Here's how the part is built. I have some questions about the finished solid (model axes, mm). A direction names the side the tool comes from. Round coordinates to 2 decimals unless told otherwise and drop trailing zeros. Loops run counter-clockwise (first coordinate to the right, second up) from the corner with the lowest first, then second, coordinate; pieces in that order, holes last. Notation, with made-up numbers: M -30.75,50 L 22.25,50 A9 ccw 22.25,60 Z; hole C -24,-38 d5. An arc over 180 degrees is marked long. Answer as a JSON object with one key per item and string values.
from build123d import *

# Parameters (mm, degrees)
SKETCH_1_W           = 15
SKETCH_1_H           = 15
EXTRUDE_1_DEPTH      = 4
EXTRUDE_2_DEPTH      = 5.5
EXTRUDE_2_DEPTH_BACK = 9.5
SKETCH_2_R           = 4.25
SKETCH_5_R           = 3
CUT_EXTRUDE_3_DEPTH  = 19.371173071
SKETCH_3_R           = 1
CUT_EXTRUDE_1_DEPTH  = 15.239030866
SKETCH_4_R           = 2
CUT_EXTRUDE_2_DEPTH  = 1
SKETCH_6_W           = 1
SKETCH_6_H           = 2.949438202
CUT_EXTRUDE_4_DEPTH  = 3.5


with BuildPart() as part:
    # 草图1 → 拉伸1 (new body)
    with BuildSketch(Plane(origin=(0, 0, 0), x_dir=(1, 0, 0), z_dir=(0, 1, 0))):
        Rectangle(SKETCH_1_W, SKETCH_1_H)
    extrude(amount=EXTRUDE_1_DEPTH)

    # 草图2 → 拉伸2 (add, two sides: drawn at the far end of the back side and taken through both)
    with BuildSketch(Plane(origin=(0, 4, 0), x_dir=(-1, 0, 0), z_dir=(0, 1, 0)).offset(-EXTRUDE_2_DEPTH_BACK)):
        with Locations(Location((0, 0, 0), (0, 0, 90))):
            Circle(SKETCH_2_R)
    extrude(amount=EXTRUDE_2_DEPTH + EXTRUDE_2_DEPTH_BACK)

    # 草图5 → 切除-拉伸3 (cut, through all)
    with BuildSketch(Plane.XZ.offset(5.5)):
        with Locations(Location((0, 0, 0), (0, 0, 270))):
            Circle(SKETCH_5_R)
    extrude(amount=-CUT_EXTRUDE_3_DEPTH, mode=Mode.SUBTRACT)

    # 草图3 → 切除-拉伸1 (cut, through all)
    with BuildSketch(Plane(origin=(0, 4, 0), x_dir=(-1, 0, 0), z_dir=(0, 1, 0))):
        with Locations(Location((5, -5, 0), (0, 0, 90))):
            Circle(SKETCH_3_R)
        with Locations(Location((-5, 5, 0), (0, 0, 90))):
            Circle(SKETCH_3_R)
    extrude(amount=-CUT_EXTRUDE_1_DEPTH, mode=Mode.SUBTRACT)

    # 草图4 → 切除-拉伸2 (cut)
    with BuildSketch(Plane(origin=(0, 4, 0), x_dir=(-1, 0, 0), z_dir=(0, 1, 0))):
        with Locations(Location((5, -5, 0), (0, 0, 90))):
            Circle(SKETCH_4_R)
        with Locations(Location((-5, 5, 0), (0, 0, 90))):
            Circle(SKETCH_4_R)
    extrude(amount=-CUT_EXTRUDE_2_DEPTH, mode=Mode.SUBTRACT)

    # 草图6 → 切除-拉伸4 (cut)
    with BuildSketch(Plane(origin=(0, 9.5, 0), x_dir=(-1, 0, 0), z_dir=(0, 1, 0))):
        with Locations((0, 3.651685393)):
            Rectangle(SKETCH_6_W, SKETCH_6_H)
    extrude(amount=-CUT_EXTRUDE_4_DEPTH, mode=Mode.SUBTRACT)


solid = part.part
Item 1: Please list where these lines run through material, in increasing order: probe 1 along X at (y, z) = (3.6, -5); probe 2 along Z at (x, y) = (0, 2.25); probe 3 along X at (y, z) = (1.8, -5). Write a range as from..to.
Resolved:
{"probe 1": "-7.5..-7, -3..7.5", "probe 2": "-7.5..-3, 3..7.5", "probe 3": "-7.5..-6, -4..7.5"}
Item 2: If we mould it in two halves opening along X, with no side actions, what happens to faces 1 (the face through (5.088, 3.507, 3.002)), 2 (the face through (7.5, 2, 0)), 3 (the face through (-1, -5.5, -3)), 4 (the face through (-0.5, 8, 4))? For each: pulls with the +X half, pulls with the -X half, needs draft (parallel to the pull), parting line crosses it, or undercut.
Resolved:
{"face 1": "undercut", "face 2": "pulls with the +X half", "face 3": "needs draft", "face 4": "undercut"}
Item 3: I want a section at B-B, the plane y = 2.5. Please give me the cut outline in (x, z), then the cut area to 3 significant figures.
Resolved:
{"outline": "M -7.5,-7.5 L 7.5,-7.5 L 7.5,7.5 L -7.5,7.5 Z; hole C -5,-5 d2; hole C 0,0 d6; hole C 5,5 d2", "area": "190 mm²"}
Item 4: I'm going to push flat-ended pins straight in: pin 1 Ø1 at (x, y) = (1, -2) entering from +Z; pin 2 Ø1.5 at (y, z) = (7, 3) entering from +X; pin 3 Ø5 at (x, z) = (-5.5, 5.5) entering from -Y; pin 4 Ø8 at (x, z) = (0, 0) entering from -Y. Where does each tip first touch, or does it pass through?
Resolved:
{"pin 1": "z = 4.22", "pin 2": "x = 3.61", "pin 3": "y = 0", "pin 4": "y = -5.5"}
Item 5: I want a section at A-A, the plane x = 0. Please give me the cut outline in (y, z).
Resolved:
{"outline": "M -5.5,-4.25 L 0,-4.25 L 0,-7.5 L 4,-7.5 L 4,-4.25 L 9.5,-4.25 L 9.5,-3 L -5.5,-3 Z; M -5.5,3 L 6,3 L 6,4.25 L 4,4.25 L 4,7.5 L 0,7.5 L 0,4.25 L -5.5,4.25 Z"}
Item 6: I want a section at C-C, the plane z = -5. Please give me the cut outline in (x, y).
Resolved:
{"outline": "M -7.5,0 L -6,0 L -6,3 L -7,3 L -7,4 L -7.5,4 Z; M -4,0 L 7.5,0 L 7.5,4 L -3,4 L -3,3 L -4,3 Z"}
Item 7: I want a section at D-D, the plane x = 5. Please give me the cut outline in (y, z).
Resolved:
{"outline": "M 0,-7.5 L 4,-7.5 L 4,3 L 3,3 L 3,4 L 0,4 Z; M 0,6 L 3,6 L 3,7 L 4,7 L 4,7.5 L 0,7.5 Z"}
Item 8: On a 3-axis mill with a long thin cutter (end or side, diameter ignored), from which of +Z, -Z, +X, -X, +Y, -Y can I reach the whole of each face in a straight line? I mean faces 5 (the face through (3, 9.5, -1)), 6 (the face through (4.214, -2.788, -0.553)), 7 (the face through (0, 6, 4)), 8 (the face through (4.214, 6.712, -0.553)). Say none if no direction works.
Resolved:
{"face 5": "+Z, -Z, +X, -X, +Y", "face 6": "-Y", "face 7": "+Z, +Y", "face 8": "+Y"}
